Design review of the part shown in the three views and the two pictorial views. Dimensions are in mm from the part's minimum x, y and z. A direction names the side the tool comes from. Round coordinates to 2 decimals unless told otherwise and drop trailing zeros. Write each loop counter-clockwise with the first axis right and the second up, starting at its lowest first coordinate (ties: lowest second). Pieces come first, ordered by that corner, then holes. Notation, with made-up numbers: (-23, 66) -> (28, 66) arc R17 cw to (28, 83) -> close; hole circle Ø1 at (35.25, 4.5). An arc over 180 degrees is marked (long way). One line per question, with ' | ' between items. Start each with the question number.
1) For the marked faces 1 and 2, list the 3-axis set-ups (+Z, -Z, +X, -X, +Y, -Y) from which the entire face can be reached by the end or side of a thin tool; tool diameter is ignored.
2) Insertion check: pin 1 Ø1 at (x, y) = (22.5, 13) entering from +Z; pin 2 Ø1 at (x, z) = (20, 1.5) entering from +Y; pin 3 Ø0.5 at (y, z) = (9.5, 1) entering from +X. Each pin has a flat end and moves straight along its axis. Give the tip position at first contact, or say it passes through.
3) Consider section C-C (x = 22). Give the boundary of the cut face in (y, z).
4) For probe 1 along Z at (x, y) = (12.25, 2.5); probe 2 along Y at (x, z) = (15.5, 1.15); probe 3 along Z at (x, y) = (8, 19.5), list the stretches that pass through material, from the lowest coordinate up.
5) Consider section A-A (z = 1.15). Give the boundary of the cut face in (x, y).
6) Consider section B-B (y = 5.5). Give the boundary of the cut face in (x, z), then the cut area to 3 significant figures.
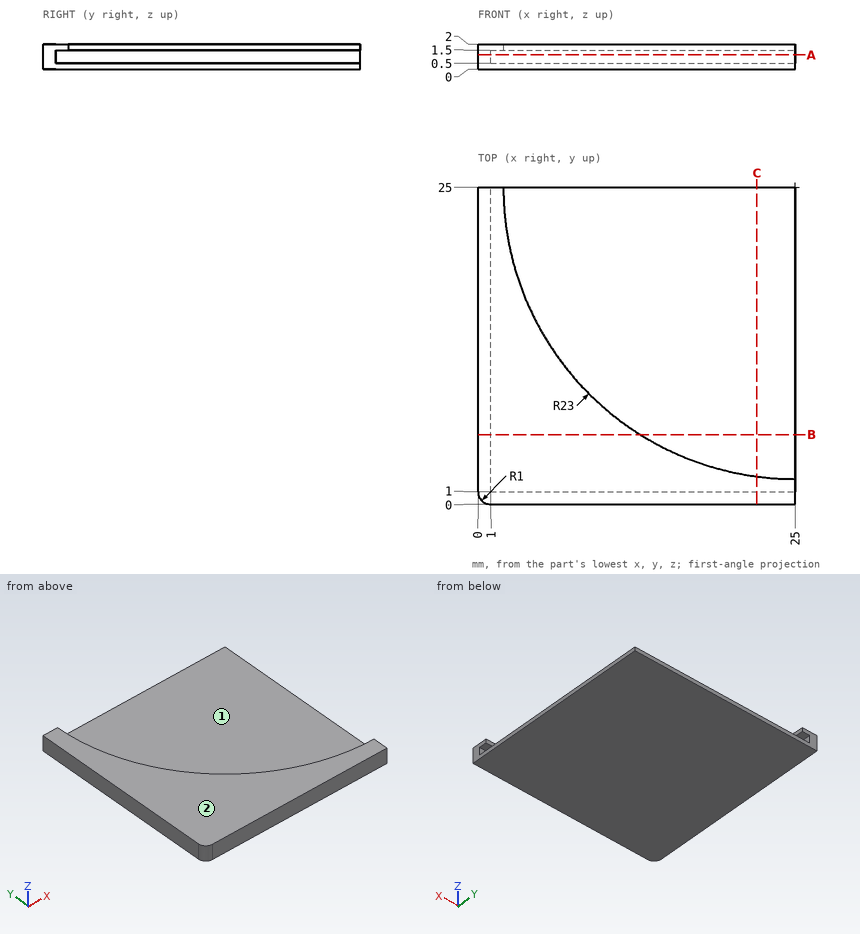
From the geometry:
1) face 1: +X, +Y | face 2: +Z, +X, -X, +Y, -Y
2) pin 1: stops at z = 0.5 | pin 2: stops at y = 2.67 | pin 3: stops at x = 1
3) outline: (0, 0) -> (25, 0) -> (25, 0.5) -> (1, 0.5) -> (1, 1.5) -> (2.2, 1.5) -> (2.2, 2) -> (0, 2) -> close
4) probe 1: z = 0 to 0.5, 1.5 to 2 | probe 2: y = 0 to 1 | probe 3: z = 0 to 0.5
5) outline: (0, 1) arc R1 ccw to (1, 0) -> (25, 0) -> (25, 1) -> (1, 1) -> (1, 25) -> (0, 25) -> close
6) outline: (0, 0) -> (25, 0) -> (25, 0.5) -> (1, 0.5) -> (1, 1.5) -> (12.8, 1.5) -> (12.8, 2) -> (0, 2) -> close | area: 19.9 mm2
